Model file for the job. Use its own axes, mm. Round coordinates to 2 decimals unless told otherwise and drop trailing zeros. Order: outer loops, then holes, each group sorted by start corner. A loop starts at its lowest first (then second) coordinate and runs counter-clockwise, first axis right, second up. Notation, with made-up numbers: (-8.75, -19) - (44.25, -19) arc R18 cw to (44.25, -6) - close; hole circle Ø3 at (67, 87.25). An arc over 180 degrees is marked (long way). Put each result on its own line as item: value. Start each with the question number.
Item 1: Saw through at A-A on x = -10. List the corners of the cut face in (y, z).
Item 2: Probe probe 1 along X at (y, z) = (-2.5, 63); probe 2 along Z at (x, y) = (80, -3); probe 3 along X at (y, z) = (-2.3, -51). List the from-to ranges inside material, lowest first.
Item 3: Saw through at B-B on x = -52.5. List the corners of the cut face in (y, z), plus the area to 3 significant figures.
Item 4: Saw through at D-D on x = 29.5. List the corners of the cut face in (y, z).
Item 5: Saw through at C-C on y = -2.6. List the corners of the cut face in (x, z).
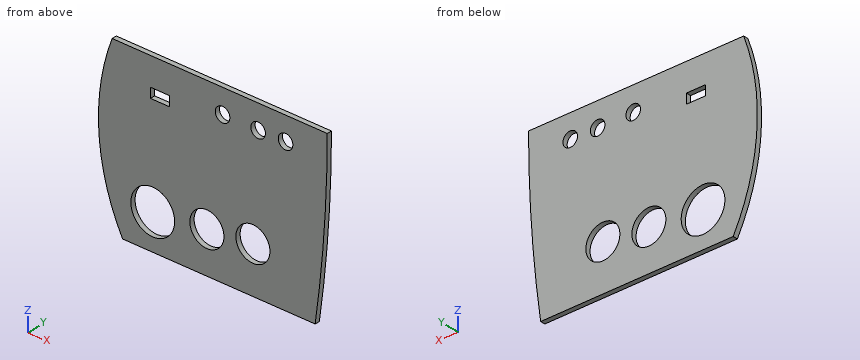
```python
from build123d import *

# Parameters (mm, degrees)
F0_R     = 22.5
F0_R_2   = 17.5
F0_W     = 19.454152
F0_H     = 10.062493
F0_R_3   = 7.5
F1_DEPTH = 5


with BuildPart() as f1:
    # F0 (on Front) → F1 (new body)
    with BuildSketch(Plane.XZ):
        with BuildLine():
            Line((-92.498694, -88.391484), (105.413623, -88.391484))
            ThreePointArc((105.413623, -88.391484), (114.741048, -0.218636), (117.855312, 88.391484))
            Line((117.855312, 88.391484), (-103.311009, 88.391484))
            ThreePointArc((-103.311009, 88.391484), (-116.943778, -1.16445), (-92.498694, -88.391484))
        make_face()
        with Locations((-61.532475, -52.015223)):
            Circle(F0_R, mode=Mode.SUBTRACT)
        with Locations((-5.853384, -45.977734)):
            Circle(F0_R_2, mode=Mode.SUBTRACT)
        with Locations((41.440301, -40.946487)):
            Circle(F0_R_2, mode=Mode.SUBTRACT)
        with Locations((-54.153323, 54.64714)):
            Rectangle(F0_W, F0_H, mode=Mode.SUBTRACT)
        with Locations((10.246594, 63.703366)):
            Circle(F0_R_3, mode=Mode.SUBTRACT)
        with Locations((46.806965, 63.703366)):
            Circle(F0_R_3, mode=Mode.SUBTRACT)
        with Locations((74.981928, 64.374208)):
            Circle(F0_R_3, mode=Mode.SUBTRACT)
    extrude(amount=F1_DEPTH)


solid = f1.part
```
Results found:
1. outline: (-5, -88.39) - (0, -88.39) - (0, -62.98) - (-5, -62.98) - close; (-5, -28.98) - (0, -28.98) - (0, 88.39) - (-5, 88.39) - close
2. probe 1: x = -111.2 to 2.78, 17.71 to 39.34, 54.27 to 67.61, 82.35 to 117.6
2. probe 2: z = -88.39 to 58.8, 69.95 to 88.39
2. probe 3: x = -107.92 to -84.01, -39.06 to -22.62, 10.91 to 27.12, 55.76 to 110.13
3. outline: (-5, -88.39) - (0, -88.39) - (0, -72.62) - (-5, -72.62) - close; (-5, -31.41) - (0, -31.41) - (0, 49.62) - (-5, 49.62) - close; (-5, 59.68) - (0, 59.68) - (0, 88.39) - (-5, 88.39) - close
3. area: 628 mm²
4. outline: (-5, -88.39) - (0, -88.39) - (0, -53.74) - (-5, -53.74) - close; (-5, -28.15) - (0, -28.15) - (0, 88.39) - (-5, 88.39) - close
5. outline: (-103.31, 88.39) arc R215.11 ccw to (-92.5, -88.39) - (105.41, -88.39) arc R1262.17 ccw to (117.86, 88.39) - close; hole circle Ø45 at (-61.53, -52.02); hole (-63.88, 49.62) - (-44.43, 49.62) - (-44.43, 59.68) - (-63.88, 59.68) - close; hole circle Ø35 at (-5.85, -45.98); hole circle Ø15 at (10.25, 63.7); hole circle Ø35 at (41.44, -40.95); hole circle Ø15 at (46.81, 63.7); hole circle Ø15 at (74.98, 64.37)
